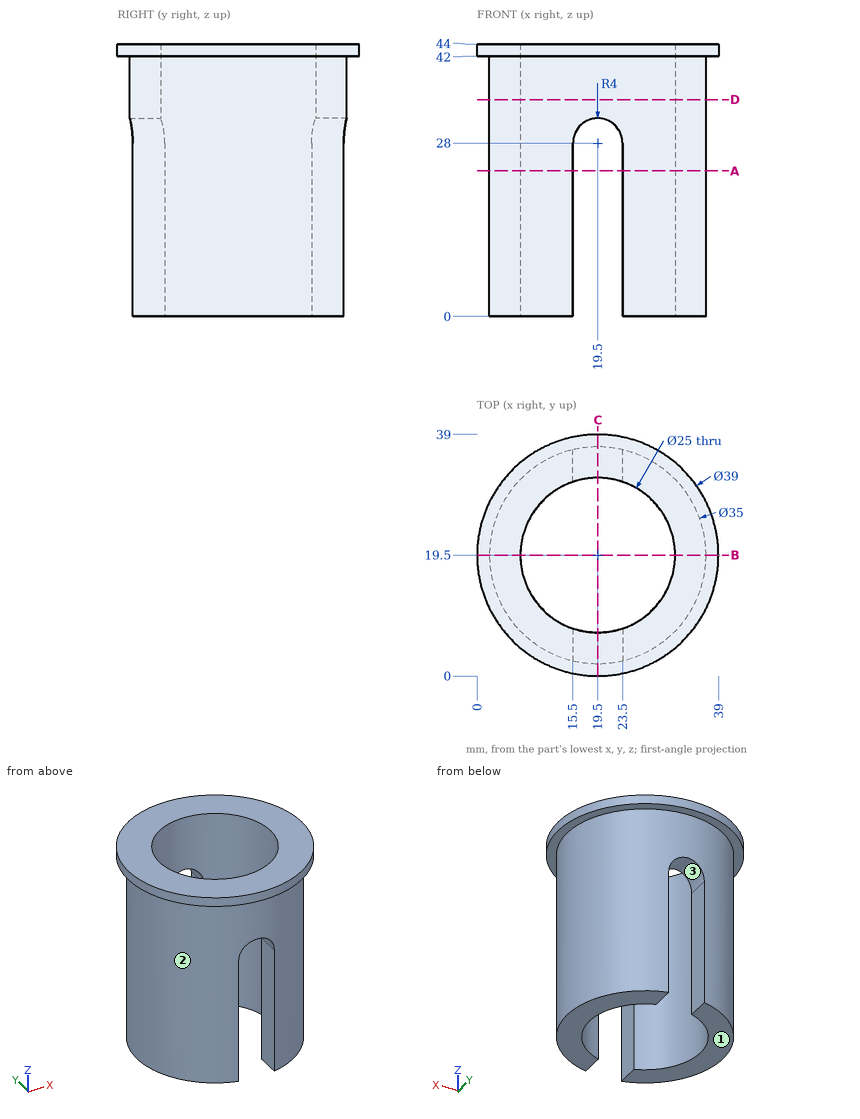
For this review, use the dimensioned drawing (mm, ordinates from the lowest corner) and the shaded views. Give positions to 0.01 mm unless a question says otherwise; leave off trailing zeros. Order: outer loops, then holes, each group sorted by start corner. A loop starts at its lowest first (then second) coordinate and runs counter-clockwise, first axis right, second up.
1) Insertion check: pin 1 (5.5 mm diameter, centred on y = 5.5, z = 13.5, fed in from -X); pin 2 (3 mm diameter, centred on y = 19.5, z = 27.5, fed in from -X); pin 3 (2.5 mm diameter, centred on y = 35, z = 17, fed in from -X); pin 4 (20 mm diameter, centred on x = 19.5, y = 19.5, fed in from +Z). Each pin has a flat end and moves straight along its axis. Give the tip position at first contact, or say it passes through.
2) Wall thickness on line 1 (X direction, y = 19, z = 24); line 2 (Y direction, x = 19.5, z = 34); line 3 (Y direction, x = 15, z = 25): over which ranges is each line inside the solid? List them lowest first.
3) Take a section at B-B (y = 19.5). Give the boundary of the cut face in (x, z), then the cut area to 3 significant figures.
4) Take a section at A-A (z = 23.5). Give the boundary of the cut face in (x, y).
5) Take a section at C-C (x = 19.5). Give the boundary of the cut face in (y, z), then the cut area to 3 significant figures.
6) The part is to be moulded in two halves that separate along X. For the marked faces 1, 2 and 3, say which applies: released by +X, released by -X, zero draft, split by the parting line, or undercut.
7) Take a section at D-D (z = 35). Give the boundary of the cut face in (x, y), then the cut area to 3 significant figures.
Derived:
1. pin 1: stops at x = 6.1
1. pin 2: stops at x = 2
1. pin 3: stops at x = 9.34
1. pin 4: passes through
2. line 1: x = 2.01 to 7.01, 31.99 to 36.99
2. line 2: y = 2 to 7, 32 to 37
2. line 3: y = 2.59 to 7.84, 31.16 to 36.41
3. outline: (0, 42) - (2, 42) - (2, 0) - (7, 0) - (7, 44) - (0, 44) - close; (32, 0) - (37, 0) - (37, 42) - (39, 42) - (39, 44) - (32, 44) - close
3. area: 448 mm2
4. outline: (15.5, 2.46) - (15.5, 7.66) arc R12.5 cw to (15.5, 31.34) - (15.5, 36.54) arc R17.5 ccw to start; (23.5, 2.46) arc R17.5 ccw to (23.5, 36.54) - (23.5, 31.34) arc R12.5 cw to (23.5, 7.66) - close
5. outline: (0, 42) - (2, 42) - (2, 32) - (7, 32) - (7, 44) - (0, 44) - close; (32, 32) - (37, 32) - (37, 42) - (39, 42) - (39, 44) - (32, 44) - close
5. area: 128 mm2
6. face 1: zero draft
6. face 2: split by the parting line
6. face 3: undercut
7. outline: circle Ø35 at (19.5, 19.5); hole circle Ø25 at (19.5, 19.5)
7. area: 471 mm2
